Verification items for the finished model (mm, model axes). A direction names the side the tool comes from. Give positions to 0.01 mm unless a question says otherwise; leave off trailing zeros. Loops run counter-clockwise (first coordinate to the right, second up) from the corner with the lowest first, then second, coordinate; pieces in that order, holes last. Notation, with made-up numbers: (-39, 18.25) - (-35, 18.25) arc R15 ccw to (-35, 23.25) - close; hole circle Ø10 at (-37.75, 21). An arc over 180 degrees is marked (long way). Answer in a Markdown table with one row per item.
```python
from build123d import *

# Parameters (mm, degrees)
SKETCH1_W               = 42
SKETCH1_H               = 42
BOSS_EXTRUDE1_DEPTH     = 17
SKETCH3_W               = 42
SKETCH3_H               = 13
CUT_EXTRUDE1_DEPTH      = 32.7
CUT_EXTRUDE2_DEPTH      = 61.802960454
CUT_EXTRUDE2_DEPTH_BACK = 61.802960454
SKETCH4_R               = 1.6
SKETCH4_R_2             = 11
SKETCH5_R               = 2.5
CUT_EXTRUDE3_DEPTH      = 2
SKETCH6_R               = 1.5
SKETCH6_R_2             = 3
CUT_EXTRUDE4_DEPTH      = 56.877455203


with BuildPart() as part:
    # Sketch1 → Boss-Extrude1 (new body)
    with BuildSketch(Plane.XY):
        with Locations((21, 21)):
            Rectangle(SKETCH1_W, SKETCH1_H)
    extrude(amount=BOSS_EXTRUDE1_DEPTH)

    # Sketch3 → Cut-Extrude1 (cut)
    with BuildSketch(Plane(origin=(0, 42, 0), x_dir=(1, 0, 0), z_dir=(0, 1, 0))):
        with Locations((21, -10.5)):
            Rectangle(SKETCH3_W, SKETCH3_H)
    extrude(amount=-CUT_EXTRUDE1_DEPTH, mode=Mode.SUBTRACT)

    # Sketch4 → Cut-Extrude2 (cut, two sides: drawn at the far end of the back side and taken through both)
    with BuildSketch(Plane.XY.offset(4).offset(-CUT_EXTRUDE2_DEPTH_BACK)):
        with Locations((36.5, 36.5)):
            Circle(SKETCH4_R)
        with Locations((5.5, 36.5)):
            Circle(SKETCH4_R)
        with Locations((21, 21)):
            Circle(SKETCH4_R_2)
        with Locations((5.5, 5.5)):
            Circle(SKETCH4_R)
        with Locations((36.5, 5.5)):
            Circle(SKETCH4_R)
    extrude(amount=CUT_EXTRUDE2_DEPTH + CUT_EXTRUDE2_DEPTH_BACK, mode=Mode.SUBTRACT)

    # Sketch5 → Cut-Extrude3 (cut)
    with BuildSketch(Plane.XY.offset(4)):
        with Locations((36.5, 36.5)):
            Circle(SKETCH5_R)
    extrude(amount=-CUT_EXTRUDE3_DEPTH, mode=Mode.SUBTRACT)

    # Sketch6 → Cut-Extrude4 (cut, through all)
    with BuildSketch(Plane(origin=(0, 9.3, 0), x_dir=(1, 0, 0), z_dir=(0, 1, 0))):
        with Locations(Location((32, -11, 0), (0, 0, 270))):
            Circle(SKETCH6_R)
        with Locations(Location((14.5, -11, 0), (0, 0, 270))):
            Circle(SKETCH6_R_2)
    extrude(amount=-CUT_EXTRUDE4_DEPTH, mode=Mode.SUBTRACT)


solid = part.part
```
Q1. Thickness scan on line 1 (Y direction, x = 36.5, z = 3.2); line 2 (Y direction, x = 36.5, z = 0.65); line 3 (Y direction, x = 21, z = 1). Record the ranges inside material, lowest first.
Completed:
| item | result |
|---|---|
| line 1 | 0 to 3.9, 7.1 to 34, 39 to 42 |
| line 2 | 0 to 3.9, 7.1 to 34.9, 38.1 to 42 |
| line 3 | 0 to 10, 32 to 42 |
Q2. Sectioned sample at A-A (y = 5.5). Record the cut outline in (x, z), and give its area (3 significant figures).
Completed:
| item | result |
|---|---|
| outline | (0, 0) - (3.9, 0) - (3.9, 17) - (0, 17) - close; (7.1, 0) - (34.9, 0) - (34.9, 17) - (7.1, 17) - close; (38.1, 0) - (42, 0) - (42, 17) - (38.1, 17) - close; hole circle Ø6 at (14.5, 11); hole circle Ø3 at (32, 11) |
| area | 570 mm^2 |
Q3. Sectioned sample at B-B (z = 11). Record the cut outline in (x, y), and give its area (3 significant figures).
Completed:
| item | result |
|---|---|
| outline | (0, 0) - (11.5, 0) - (11.5, 9.3) - (0, 9.3) - close; (17.5, 0) - (30.5, 0) - (30.5, 9.3) - (17.5, 9.3) - close; (33.5, 0) - (42, 0) - (42, 9.3) - (33.5, 9.3) - close; hole circle Ø3.2 at (5.5, 5.5); hole circle Ø3.2 at (36.5, 5.5) |
| area | 291 mm^2 |
Q4. Go/stop test with flat-tipped pins: P1, Ø5, axis at x = 14, y = 30, coming from the +Z side; P2, Ø3.5, axis at x = 5.5, y = 36.5, coming from the -Z side; P3, Ø2.5, axis at x = 36.5, y = 5.5, coming from the +Z side; P4, Ø6, axis at x = 27, z = 15, coming from the +Y side. Record where each tip stops, or that it passes through.
Completed:
| item | result |
|---|---|
| P1 | z = 4 |
| P2 | z = 0 |
| P3 | through |
| P4 | y = 9.3 |
Q5. Tool access check on faces 1 (the face through (35, 38, 2)), 2 (the face through (30, 12, 0)). Record the directions out of +Z, -Z, +X, -X, +Y, -Y that give a thin tool (end or side, any length) a straight path to the whole face; none if there is none.
Completed:
| item | result |
|---|---|
| face 1 | +Z |
| face 2 | -Z, +X, -X, +Y, -Y |
Q6. Draft check along Y on faces 3 (the face through (37.24, 35.08, 0.99)), 4 (the face through (21, 9.3, 10)), 5 (the face through (21, 33, 4)). Enter one of: +Y half, -Y half, draft (parallel to the pull), parting line (faces both ways), or undercut.
Completed:
| item | result |
|---|---|
| face 3 | undercut |
| face 4 | +Y half |
| face 5 | draft |
Q7. Sectioned sample at C-C (x = 36.5). Record the cut outline in (y, z), and give its area (3 significant figures).
Completed:
| item | result |
|---|---|
| outline | (0, 0) - (3.9, 0) - (3.9, 17) - (0, 17) - close; (7.1, 0) - (34.9, 0) - (34.9, 2) - (34, 2) - (34, 4) - (9.3, 4) - (9.3, 17) - (7.1, 17) - close; (38.1, 0) - (42, 0) - (42, 4) - (39, 4) - (39, 2) - (38.1, 2) - close |
| area | 218 mm^2 |
Q8. Sectioned sample at D-D (y = 21). Record the cut outline in (x, z), and give its area (3 significant figures).
Completed:
| item | result |
|---|---|
| outline | (0, 0) - (10, 0) - (10, 4) - (0, 4) - close; (32, 0) - (42, 0) - (42, 4) - (32, 4) - close |
| area | 80.0 mm^2 |
